For this review, take the finished solid that the model builds, in its own axes (mm). A direction names the side the tool comes from. Coordinates: 2 decimals unless noted, no trailing zeros. Write each loop counter-clockwise with the first axis right and the second up, starting at its lowest first coordinate (ties: lowest second). Pieces come first, ordered by that corner, then holes.
```python
from build123d import *

# Parameters (mm, degrees)
SKETCH1_W           = 45
SKETCH1_H           = 45
BOSS_EXTRUDE1_DEPTH = 14
CUT_EXTRUDE1_DEPTH  = 35.763486592
CHAMFER1_SIZE       = 0.5
CHAMFER2_SIZE       = 2
SKETCH4_R           = 1.75
CUT_EXTRUDE2_DEPTH  = 35.763486592
SKETCH5_R           = 1.75
SKETCH5_W           = 41
SKETCH5_H           = 2
SKETCH5_W_2         = 2
SKETCH5_H_2         = 41
BOSS_EXTRUDE3_DEPTH = 5
SKETCH6_R           = 1.75
BOSS_EXTRUDE4_DEPTH = 19
REVOLVE4_OUTLINE_R  = 2.5
REVOLVE4_ANGLE      = 180


# Read off the part's stored shape, not the designer's step: Revolve4
with BuildPart() as part:
    # Sketch1 → Boss-Extrude1 (new body)
    with BuildSketch(Plane(origin=(0, 0, 0), x_dir=(1, 0, 0), z_dir=(0, 1, 0))):
        Rectangle(SKETCH1_W, SKETCH1_H)
    extrude(amount=BOSS_EXTRUDE1_DEPTH)

    # Sketch3 → Cut-Extrude1 (cut, through all)
    with BuildSketch(Plane(origin=(0, 14, 0), x_dir=(1, 0, 0), z_dir=(0, 1, 0))):
        with BuildLine():
            Line((-22.5, 12.75), (-8.05, 12.75))
            ThreePointArc((-8.05, 12.75), (-6.211522369, 13.511522369), (-5.45, 15.35))
            Line((-5.45, 15.35), (-5.45, 16.35))
            ThreePointArc((-5.45, 16.35), (-4.688477631, 18.188477631), (-2.85, 18.95))
            Line((-2.85, 18.95), (2.65, 18.95))
            ThreePointArc((2.65, 18.95), (4.488477631, 18.188477631), (5.25, 16.35))
            Line((5.25, 16.35), (5.25, 15.35))
            ThreePointArc((5.25, 15.35), (6.011522369, 13.511522369), (7.85, 12.75))
            Line((7.85, 12.75), (16.5, 12.75))
            Line((16.5, 12.75), (16.5, -12.75))
            Line((16.5, -12.75), (7.85, -12.75))
            ThreePointArc((7.85, -12.75), (6.011522369, -13.511522369), (5.25, -15.35))
            Line((5.25, -15.35), (5.25, -16.35))
            ThreePointArc((5.25, -16.35), (4.488477631, -18.188477631), (2.65, -18.95))
            Line((2.65, -18.95), (-2.85, -18.95))
            ThreePointArc((-2.85, -18.95), (-4.688477631, -18.188477631), (-5.45, -16.35))
            Line((-5.45, -16.35), (-5.45, -15.35))
            ThreePointArc((-5.45, -15.35), (-6.211522369, -13.511522369), (-8.05, -12.75))
            Line((-8.05, -12.75), (-22.5, -12.75))
            Line((-22.5, -12.75), (-22.5, 12.75))
        make_face()
    extrude(amount=-CUT_EXTRUDE1_DEPTH, mode=Mode.SUBTRACT)

    # Chamfer1
    chamfer1_edges = [part.edges().sort_by_distance(p)[0] for p in [
        (-22.5, 14, -17.625),
        (0, 14, 22.5),
        (-22.5, 14, 17.625),
        (22.5, 14, 0),
        (0, 14, -22.5),
    ]]
    chamfer(chamfer1_edges, length=CHAMFER1_SIZE)

    # Chamfer2
    # the kernel refuses this chamfer: 5.464101615, 2 mm, written as the material it takes off along each edge
    # the kernel refuses this chamfer: 5.464101615, 2 mm, written as the material it takes off along each edge
    with BuildSketch(Plane(origin=(-22.5, -5.143365976, -22.5), x_dir=(-0.027495876610585647, 0, 0.9996219169112968), z_dir=(0, 1, 0)), Plane(origin=(-22.5, -5.143365976, 22.5), x_dir=(0.9996219169112968, 0, 0.027495876610585647), z_dir=(0, 1, 0))) as chamfer2_2_piece_1:
        Polygon((CHAMFER2_SIZE * 0.999621916911, CHAMFER2_SIZE * 0.0274958766106), (-CHAMFER2_SIZE * 0.0274958766106, CHAMFER2_SIZE * 0.999621916911), (0, 0), align=None)
    extrude(amount=23.786731952, mode=Mode.SUBTRACT)
    with BuildSketch(Plane(origin=(22.5, -5.143365976, 22.5), x_dir=(-0.9996219169112968, 0, 0.027495876610585647), z_dir=(0, 1, 0)), Plane(origin=(22.5, -5.143365976, -22.5), x_dir=(0.027495876610585647, 0, 0.9996219169112968), z_dir=(0, 1, 0))) as chamfer2_2_piece_2:
        Polygon((CHAMFER2_SIZE * 0.999621916911, -CHAMFER2_SIZE * 0.0274958766106), (-CHAMFER2_SIZE * 0.0274958766106, -CHAMFER2_SIZE * 0.999621916911), (0, 0), align=None)
    extrude(amount=23.786731952, mode=Mode.SUBTRACT)

    # Sketch4 → Cut-Extrude2 (cut, through all)
    with BuildSketch(Plane(origin=(0, 14, 0), x_dir=(1, 0, 0), z_dir=(0, 1, 0))):
        with Locations(Location((-18, 17.25, 0), (0, 0, 270))):
            Circle(SKETCH4_R)
        with Locations(Location((18, 17.25, 0), (0, 0, 270))):
            Circle(SKETCH4_R)
        with Locations(Location((18, -17.25, 0), (0, 0, 270))):
            Circle(SKETCH4_R)
        with Locations(Location((-18, -17.25, 0), (0, 0, 270))):
            Circle(SKETCH4_R)
    extrude(amount=-CUT_EXTRUDE2_DEPTH, mode=Mode.SUBTRACT)

    # Sketch5 → Boss-Extrude3 (add)
    # profile 1 of 7: a face of its own
    with BuildSketch(Plane.XZ):
        with BuildLine():
            Line((20.5, 20.5), (20.5, -22.5))
            Line((20.5, -22.5), (-20.5, -22.5))
            Line((-20.5, -22.5), (-22.5, -20.5))
            Line((-22.5, -20.5), (-22.5, -12.75))
            Line((-22.5, -12.75), (-8.05, -12.75))
            ThreePointArc((-8.05, -12.75), (-6.211522369, -13.511522369), (-5.45, -15.35))
            Line((-5.45, -15.35), (-5.45, -16.35))
            ThreePointArc((-5.45, -16.35), (-4.688477631, -18.188477631), (-2.85, -18.95))
            Line((-2.85, -18.95), (2.65, -18.95))
            ThreePointArc((2.65, -18.95), (4.488477631, -18.188477631), (5.25, -16.35))
            Line((5.25, -16.35), (5.25, -15.35))
            ThreePointArc((5.25, -15.35), (6.011522369, -13.511522369), (7.85, -12.75))
            Line((7.85, -12.75), (16.5, -12.75))
            Line((16.5, -12.75), (16.5, 12.75))
            Line((16.5, 12.75), (7.85, 12.75))
            ThreePointArc((7.85, 12.75), (6.011522369, 13.511522369), (5.25, 15.35))
            Line((5.25, 15.35), (5.25, 16.35))
            ThreePointArc((5.25, 16.35), (4.488477631, 18.188477631), (2.65, 18.95))
            Line((2.65, 18.95), (-2.85, 18.95))
            ThreePointArc((-2.85, 18.95), (-4.688477631, 18.188477631), (-5.45, 16.35))
            Line((-5.45, 16.35), (-5.45, 15.35))
            ThreePointArc((-5.45, 15.35), (-6.211522369, 13.511522369), (-8.05, 12.75))
            Line((-8.05, 12.75), (-22.5, 12.75))
            Line((-22.5, 12.75), (-22.5, 20.5))
            Line((-22.5, 20.5), (20.5, 20.5))
        make_face()
        with Locations(Location((18, 17.25, 0), (0, 0, 90))):
            Circle(SKETCH5_R, mode=Mode.SUBTRACT)
        with Locations(Location((-18, -17.25, 0), (0, 0, 90))):
            Circle(SKETCH5_R, mode=Mode.SUBTRACT)
        with Locations(Location((18, -17.25, 0), (0, 0, 90))):
            Circle(SKETCH5_R, mode=Mode.SUBTRACT)
        with Locations(Location((-18, 17.25, 0), (0, 0, 90))):
            Circle(SKETCH5_R, mode=Mode.SUBTRACT)
    # profile 2 of 7: a face of its own
    with BuildSketch(Plane.XZ):
        with Locations((0, 21.5)):
            Rectangle(SKETCH5_W, SKETCH5_H)
    # profile 3 of 7: a face of its own
    with BuildSketch(Plane.XZ):
        Polygon((-22.5, 20.5), (-20.5, 20.5), (-20.5, 22.5), align=None)
    # profile 4 of 7: a face of its own
    with BuildSketch(Plane.XZ):
        Polygon((22.5, 20.5), (20.5, 20.5), (20.5, 22.5), align=None)
    # profile 5 of 7: a face of its own
    with BuildSketch(Plane.XZ):
        with Locations((21.5, 0)):
            Rectangle(SKETCH5_W_2, SKETCH5_H_2)
    # profile 6 of 7: a face of its own
    with BuildSketch(Plane.XZ):
        Polygon((20.5, -20.5), (20.5, -22.5), (22.5, -20.5), align=None)
    # profile 7 of 7: a face of its own
    with BuildSketch(Plane.XZ):
        with BuildLine():
            Line((-22.5, 12.75), (-22.5, -12.75))
            Line((-22.5, -12.75), (-8.05, -12.75))
            ThreePointArc((-8.05, -12.75), (-6.211522369, -13.511522369), (-5.45, -15.35))
            Line((-5.45, -15.35), (-5.45, -16.35))
            ThreePointArc((-5.45, -16.35), (-4.688477631, -18.188477631), (-2.85, -18.95))
            Line((-2.85, -18.95), (2.65, -18.95))
            ThreePointArc((2.65, -18.95), (4.488477631, -18.188477631), (5.25, -16.35))
            Line((5.25, -16.35), (5.25, -15.35))
            ThreePointArc((5.25, -15.35), (6.011522369, -13.511522369), (7.85, -12.75))
            Line((7.85, -12.75), (16.5, -12.75))
            Line((16.5, -12.75), (16.5, 12.75))
            Line((16.5, 12.75), (7.85, 12.75))
            ThreePointArc((7.85, 12.75), (6.011522369, 13.511522369), (5.25, 15.35))
            Line((5.25, 15.35), (5.25, 16.35))
            ThreePointArc((5.25, 16.35), (4.488477631, 18.188477631), (2.65, 18.95))
            Line((2.65, 18.95), (-2.85, 18.95))
            ThreePointArc((-2.85, 18.95), (-4.688477631, 18.188477631), (-5.45, 16.35))
            Line((-5.45, 16.35), (-5.45, 15.35))
            ThreePointArc((-5.45, 15.35), (-6.211522369, 13.511522369), (-8.05, 12.75))
            Line((-8.05, 12.75), (-22.5, 12.75))
        make_face()
    extrude(amount=BOSS_EXTRUDE3_DEPTH)

    # Sketch6 → Boss-Extrude4 (add)
    with BuildSketch(Plane(origin=(0, 14, 0), x_dir=(1, 0, 0), z_dir=(0, 1, 0))):
        with Locations((-18, 17.25)):
            Circle(SKETCH6_R)
        with Locations((18, 17.25)):
            Circle(SKETCH6_R)
        with Locations((-18, -17.25)):
            Circle(SKETCH6_R)
        with Locations((18, -17.25)):
            Circle(SKETCH6_R)
    extrude(amount=-BOSS_EXTRUDE4_DEPTH)

    # Revolve4 outline → Revolve4 (revolve)
    with BuildSketch(Plane(origin=(0, 0, 22.5), x_dir=(-1, 0, 0), z_dir=(0, 0, -1))):
        with Locations((15.5, 4.5)):
            Circle(REVOLVE4_OUTLINE_R)
    revolve4 = revolve(axis=Axis((0, 0, 22.5), (0, 1, 0)), revolution_arc=REVOLVE4_ANGLE)

    # Mirror1: Revolve4 across plane
    add(revolve4.mirror(Plane.XY))


solid = part.part
```
Q1. Add section A-A (y = -3). State the section outline as (x, z) points, then the cut area to 3 significant figures.
Ans:
outline: (-22.5, -20.5) - (-20.5, -22.5) - (20.5, -22.5) - (22.5, -20.5) - (22.5, 20.5) - (20.5, 22.5) - (-20.5, 22.5) - (-22.5, 20.5) - close
area: 2,020 mm2
Q2. Draft analysis for pull direction Z (two halves, no side actions). For faces 1 (the flat face through (-21, 5, 22)), 2 (the flat face through (21, 5, -22)), 3 (the cylindrical face through (-4.668, 7.098, 18.209)), 4 (the cylindrical face through (-6.232, 7.098, -13.491)), state which applies: +Z half, -Z half, draft (parallel to the pull), parting line (faces both ways), or undercut.
Ans:
face 1: +Z half
face 2: -Z half
face 3: undercut
face 4: undercut
Q3. Clearance check with flat-ended pins moving along their axes: pin 1 Ø5 at (y, z) = (2.5, 31.5) entering from +X; pin 2 Ø1 at (y, z) = (7, 22.5) entering from -X; pin 3 Ø3 at (x, y) = (0, 6.5) entering from -Z. State where each tip first meets the part, or that it passes through.
Ans:
pin 1: stops at x = 16.53
pin 2: stops at x = -21
pin 3: stops at z = -40.45
Q4. Tool access review of faces 5 (the flat face through (12, 7, 12.75)), 6 (the flat face through (0, 7, 18.95)), 7 (the flat face through (0, 4, -22.5)): name each direction out of +Z, -Z, +X, -X, +Y, -Y from which nothing blocks a thin tool from reaching the whole face with its end or side.
Ans:
face 5: -X, +Y
face 6: +Y
face 7: none
Q5. Add section D-D (x = 9). Give the number of separate pieces and of enclosed holes in the cut face, then the cut area to 3 significant figures.
Ans:
separate pieces: 3
enclosed holes: 0
area: 546 mm2
Q6. For probe 1 along Z at (x, y) = (-3, 3); probe 2 along Z at (x, y) = (1.5, 12); probe 3 along Z at (x, y) = (-11.5, 11.75), list the stretches that pass through material, from the lowest coordinate up.
Ans:
probe 1: z = -39.74 to -35.66, -22.5 to -18.95, 18.95 to 22.5, 35.66 to 39.74
probe 2: z = -22.5 to -18.95, 18.95 to 22.5
probe 3: z = -22.5 to -12.75, 12.75 to 22.5
Q7. Add section B-B (z = -2.5). State the section outline as (x, y) points, then the cut area to 3 significant figures.
Ans:
outline: (-22.5, -5) - (22.5, -5) - (22.5, 13.5) - (22, 14) - (16.5, 14) - (16.5, 0) - (-22.5, 0) - close
area: 309 mm2
Q8. Add section C-C (x = 19). State the section outline as (y, z) points, then the cut area to 3 significant figures.
Ans:
outline: (-5, -22.5) - (13.5, -22.5) - (14, -22) - (14, 22) - (13.5, 22.5) - (-5, 22.5) - close
area: 855 mm2
